Can you work these out from the drawing? Everything is in mm from the part's minimum corner. A direction names the side the tool comes from. Round coordinates to 2 decimals unless told otherwise and drop trailing zeros. Write each loop counter-clockwise with the first axis right and the second up, starting at its lowest first coordinate (ties: lowest second). Pieces come first, ordered by that corner, then holes. Notation, with made-up numbers: (14, -17) - (70, -17) arc R17 cw to (70, 7) - close; hole circle Ø7 at (85, 29). An arc over 180 degrees is marked (long way). Write each question's results on one line, items separated by ' | '. Start each with the question number.
(1) Thinking about a two-plate mould opening in Y: for the marked faces 1, 2 and 3, which applies, +Y half, -Y half, draft (parallel to the pull), parting line (faces both ways), or undercut?
(2) Imagine slicing it at A-A on z = 40. Write out the boundary of the cut face in (x, y) (1 decimal), then the cut area to 3 significant figures.
(3) Imagine slicing it at C-C on z = 49. Write out the boundary of the cut face in (x, y) (1 decimal), then the cut area to 3 significant figures.
(4) On a 3-axis mill with a long thin cutter (end or side, diameter ignored), from which of +Z, -Z, +X, -X, +Y, -Y can I reach the whole of each face in a straight line? I mean the marked faces 4 and 5. Say none if no direction works.
(5) Please list where these lines run through material, in increasing order: line 1 (X direction, y = 29, z = 75.5); line 2 (Y direction, x = 21, z = 43) (1 decimal); line 3 (Y direction, x = 53, z = 35.5) (1 decimal). Write a range as [from, to].
(6) Imagine slicing it at D-D on y = 69. Write out the boundary of the cut face in (x, z).
(7) For P1, Ø10, axis at x = 42.5, z = 64.5, coming from the +Y side; P2, Ø12, axis at x = 37.5, y = 66.5, coming from the +Z side; P3, Ø3, axis at x = 42, y = 51.5, coming from the -Z side, each with a flat end and sliding along its axis, tell me the tip position at first contact or that it passes through.
(8) Imagine slicing it at B-B on x = 49. Write out the boundary of the cut face in (y, z) (1 decimal).
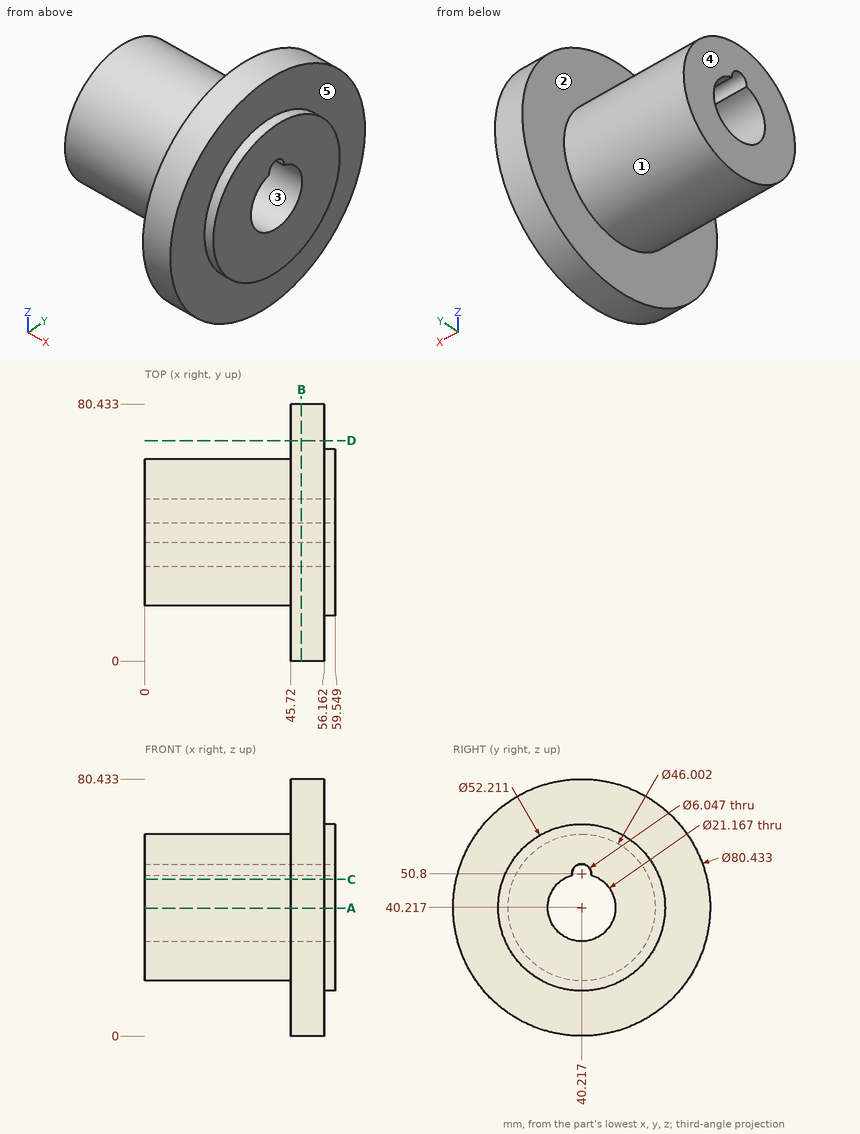
Response:
1) face 1: parting line | face 2: draft | face 3: undercut
2) outline: (0, 17.2) - (45.7, 17.2) - (45.7, 0) - (56.2, 0) - (56.2, 14.1) - (59.5, 14.1) - (59.5, 29.6) - (0, 29.6) - close; (0, 50.8) - (59.5, 50.8) - (59.5, 66.3) - (56.2, 66.3) - (56.2, 80.4) - (45.7, 80.4) - (45.7, 63.2) - (0, 63.2) - close | area: 1,860 mm²
3) outline: (0, 19) - (45.7, 19) - (45.7, 1) - (56.2, 1) - (56.2, 15.6) - (59.5, 15.6) - (59.5, 34.3) - (0, 34.3) - close; (0, 46.1) - (59.5, 46.1) - (59.5, 64.8) - (56.2, 64.8) - (56.2, 79.5) - (45.7, 79.5) - (45.7, 61.5) - (0, 61.5) - close | area: 2,230 mm²
4) face 4: +Z, -Z, -X, +Y, -Y | face 5: +X
5) line 1: [45.72, 56.16] | line 2: [17.4, 30], [50.4, 63] | line 3: [0.3, 30.7], [49.7, 80.2]
6) outline: (45.72, 12.13) - (56.16, 12.13) - (56.16, 68.3) - (45.72, 68.3) - close
7) P1: y = 74.84 | P2: z = 51.06 | P3: z = 19.4
8) outline: circle Ø80.4 at (40.2, 40.2); hole (37.2, 50.4) arc R10.6 ccw (long way) to (43.2, 50.4) arc R3 ccw (long way) to start
